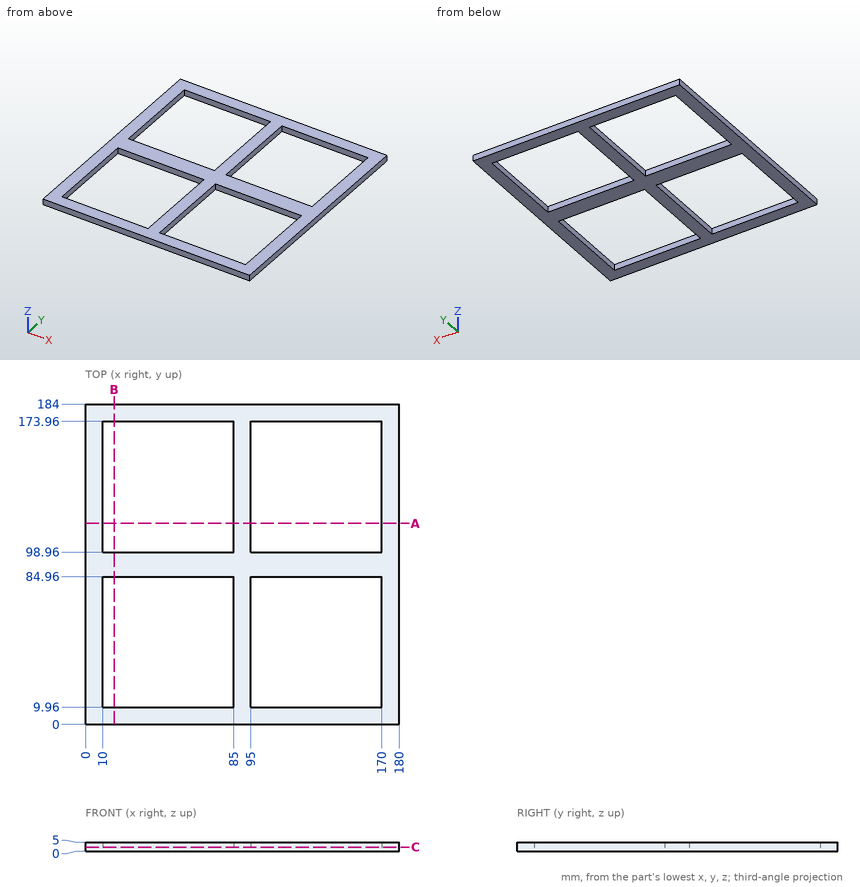
The drawing under review shows one solid part. Ordinate dimensions are in mm from its lowest x, y, z. Give positions to 0.01 mm unless a question says otherwise; leave off trailing zeros. Write each loop counter-clockwise with the first axis right and the second up, starting at its lowest first coordinate (ties: lowest second). Pieces come first, ordered by that corner, then holes.
1. Add section C-C, the plane z = 2.35. Write out the cut boundary in (x, y).
2. Add section A-A, the plane y = 115.5. Write out the cut boundary in (x, z).
3. Wall thickness on L1, parallel to Y at x = 99, z = 0.5; L2, parallel to X at y = 71, z = 1.9: over which ranges is each line inside the solid? List them lowest first.
4. Add section B-B, the plane x = 16.5. Write out the cut boundary in (y, z), plus the area to 3 significant figures.
Worked answers:
1. outline: (0, 0) - (180, 0) - (180, 184) - (0, 184) - close; hole (10, 9.96) - (85, 9.96) - (85, 84.96) - (10, 84.96) - close; hole (10, 98.96) - (85, 98.96) - (85, 173.96) - (10, 173.96) - close; hole (95, 9.96) - (170, 9.96) - (170, 84.96) - (95, 84.96) - close; hole (95, 98.96) - (170, 98.96) - (170, 173.96) - (95, 173.96) - close
2. outline: (0, 0) - (10, 0) - (10, 5) - (0, 5) - close; (85, 0) - (95, 0) - (95, 5) - (85, 5) - close; (170, 0) - (180, 0) - (180, 5) - (170, 5) - close
3. L1: y = 0 to 9.96, 84.96 to 98.96, 173.96 to 184
3. L2: x = 0 to 10, 85 to 95, 170 to 180
4. outline: (0, 0) - (9.96, 0) - (9.96, 5) - (0, 5) - close; (84.96, 0) - (98.96, 0) - (98.96, 5) - (84.96, 5) - close; (173.96, 0) - (184, 0) - (184, 5) - (173.96, 5) - close
4. area: 170 mm2
